```python
from build123d import *

# Parameters (mm, degrees)
SKETCH1_R                 = 2.15
BOSS_EXTRUDE1_DEPTH       = 6
SKETCH2_R                 = 2.15
SKETCH2_R_2               = 1
CUT_EXTRUDE1_DEPTH        = 2.5
M2X0_4_TAPPED_HOLE1_D     = 1.6
M2X0_4_TAPPED_HOLE1_DEPTH = 3.5
M2X0_4_TAPPED_HOLE1_TIP   = 0.480688495


with BuildPart() as part:
    # Sketch1 → Boss-Extrude1 (new body)
    with BuildSketch(Plane(origin=(0, 0, 0), x_dir=(1, 0, 0), z_dir=(0, 1, 0))):
        Circle(SKETCH1_R)
    extrude(amount=BOSS_EXTRUDE1_DEPTH)

    # Sketch2 → Cut-Extrude1 (cut)
    with BuildSketch(Plane(origin=(0, 6, 0), x_dir=(1, 0, 0), z_dir=(0, 1, 0))):
        Circle(SKETCH2_R)
        Circle(SKETCH2_R_2, mode=Mode.SUBTRACT)
    extrude(amount=-CUT_EXTRUDE1_DEPTH, mode=Mode.SUBTRACT)

    # M2x0.4 Tapped Hole1
    with Locations(Plane.XZ):
        with Locations((0, 0)):
            Hole(M2X0_4_TAPPED_HOLE1_D / 2, depth=M2X0_4_TAPPED_HOLE1_DEPTH)
            with Locations((0, 0, -(M2X0_4_TAPPED_HOLE1_DEPTH + M2X0_4_TAPPED_HOLE1_TIP / 2))):  # 118° drill point
                Cone(0, M2X0_4_TAPPED_HOLE1_D / 2, M2X0_4_TAPPED_HOLE1_TIP, mode=Mode.SUBTRACT)


solid = part.part
```
Source: CAD feature listing. Evaluate the final solid. Frame: model axes, mm. A direction names the side the tool comes from. Give positions to 0.01 mm unless a question says otherwise; leave off trailing zeros. Order: outer loops, then holes, each group sorted by start corner. A loop starts at its lowest first (then second) coordinate and runs counter-clockwise, first axis right, second up. Notation, with made-up numbers: (75.5, 78.5) -> (113.5, 78.5) arc R17 cw to (113.5, 88.5) -> close; hole circle Ø10 at (-14.5, -17). An arc over 180 degrees is marked (long way). Use a Markdown table: item, result.
Q1. Section B-B (x = -1.55). Return the cut outline in (y, z), and give its area (3 significant figures).
A:
| item | result |
|---|---|
| outline | (0, -1.49) -> (3.5, -1.49) -> (3.5, 1.49) -> (0, 1.49) -> close |
| area | 10.4 mm^2 |
Q2. Material intervals for line 1 (X direction, y = 1.35, z = 0); line 2 (Y direction, x = 1.05, z = -0.45), sorted ascending. Write a range as [from, to].
A:
| item | result |
|---|---|
| line 1 | [-2.15, -0.8], [0.8, 2.15] |
| line 2 | [0, 3.5] |
Q3. Section A-A (y = 3.3). Return the cut outline in (x, z), and give its area (3 significant figures).
A:
| item | result |
|---|---|
| outline | circle Ø4.3 at (0, 0); hole circle Ø1.6 at (0, 0) |
| area | 12.5 mm^2 |
Q4. Pull-direction query (Z, two-part tool) for faces 4 (the face through (0, 5, 1)), 5 (the face through (-0.139, 3.897, 0.006)), 6 (the face through (0, 0, 1)); classes: +Z half, -Z half, draft (parallel to the pull), parting line (faces both ways), or undercut.
A:
| item | result |
|---|---|
| face 4 | parting line |
| face 5 | undercut |
| face 6 | draft |
Q5. Access query for faces 1 (the face through (-1, 3.5, 1)), 2 (the face through (-2.15, 1.73, -0.09)), 3 (the face through (0.63, 1.77, -0.49)). Directions: +Z, -Z, +X, -X, +Y, -Y. A direction counts if a zero-diameter tool reaches every point of the face in a straight line with its end or side. Return the directions, or none.
A:
| item | result |
|---|---|
| face 1 | +Y |
| face 2 | +Y, -Y |
| face 3 | -Y |
Q6. First-contact query: P1, Ø1, axis at x = -1.5, z = -0.5, coming from the -Y side; P2, Ø2, axis at y = 4, z = 1.5, coming from the -X side; P3, Ø1.5, axis at x = 1.5, z = -1.5, coming from the +Y side; P4, Ø1.5, axis at y = 4.5, z = -1, coming from the -X side. Flat tips, straight axial feed; report the tip coordinate or a pass-through.
A:
| item | result |
|---|---|
| P1 | y = 0 |
| P2 | x = -2.05 |
| P3 | y = 3.5 |
| P4 | x = -0.97 |
Q7. Section D-D (z = 1.55). Return the cut outline in (x, y), and give its area (3 significant figures).
A:
| item | result |
|---|---|
| outline | (-1.49, 0) -> (1.49, 0) -> (1.49, 3.5) -> (-1.49, 3.5) -> close |
| area | 10.4 mm^2 |
Q8. Section C-C (y = 4.4). Return the cut outline in (x, z), and give its area (3 significant figures).
A:
| item | result |
|---|---|
| outline | circle Ø2 at (0, 0) |
| area | 3.14 mm^2 |
